```python
from build123d import *

# Parameters (mm, degrees)
SKETCH1_W           = 50.8
SKETCH1_H           = 25.4
SKETCH1_W_2         = 44.45
SKETCH1_H_2         = 19.05
BOSS_EXTRUDE1_DEPTH = 355.6
SKETCH2_R           = 3.3734375
CUT_EXTRUDE1_DEPTH  = 361.10715072


with BuildPart() as part:
    # Sketch1 → Boss-Extrude1 (new body)
    with BuildSketch(Plane(origin=(0, 0, 0), x_dir=(1, 0, 0), z_dir=(0, 1, 0))):
        with Locations((25.4, 12.7)):
            Rectangle(SKETCH1_W, SKETCH1_H)
        with Locations((25.4, 12.7)):
            Rectangle(SKETCH1_W_2, SKETCH1_H_2, mode=Mode.SUBTRACT)
    extrude(amount=BOSS_EXTRUDE1_DEPTH)

    # Sketch2 → Cut-Extrude1 (cut, through all)
    with BuildSketch(Plane(origin=(50.8, 0, 0), x_dir=(0, 0, -1), z_dir=(1, 0, 0))):
        with Locations((12.7, 12.7)):
            Circle(SKETCH2_R)
    cut_extrude1 = extrude(amount=-CUT_EXTRUDE1_DEPTH, mode=Mode.SUBTRACT)

    # Mirror1: Cut-Extrude1 across plane
    add(cut_extrude1.mirror(Plane.ZX.offset(177.8)), mode=Mode.SUBTRACT)


solid = part.part
```
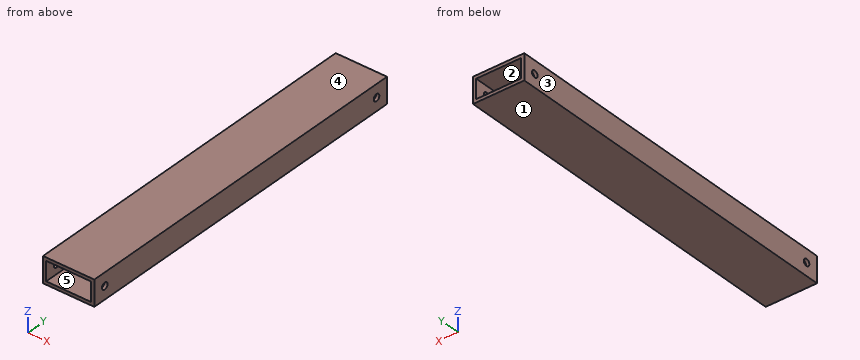
Check sheet for the modelled part. Datum: model origin and axes. Units: mm. Face numbers are marked on the shaded views. A direction names the side the tool comes from. Round coordinates to 2 decimals unless told otherwise and drop trailing zeros. Order: outer loops, then holes, each group sorted by start corner. A loop starts at its lowest first (then second) coordinate and runs counter-clockwise, first axis right, second up. Notation, with made-up numbers: (32.25, -18.5) - (81.25, -18.5) arc R22 cw to (81.25, -11.5) - close; hole circle Ø9 at (6.5, 19.5). An arc over 180 degrees is marked (long way). Answer as CSV lines item,"result". Start each with the question number.
1) Section check C-C (x = 22). Record the cut outline in (y, z) (3 decimals), then the cut area to 3 significant figures.
2) Scan lines: probe 1 along Y at (x, z) = (2, -12.7); probe 2 along X at (y, z) = (308, -11.5) (3 decimals); probe 3 along Z at (x, y) = (13.5, 321.5) (3 decimals). Record each from-to range of solid material in increasing order.
3) Tool access check on the marked faces 1 and 2. Record the directions out of +Z, -Z, +X, -X, +Y, -Y that give a thin tool (end or side, any length) a straight path to the whole face; none if there is none.
4) Section check B-B (z = -12.7). Record the cut outline in (x, y) (3 decimals).
5) Section check A-A (y = 12.7). Record the cut outline in (x, z) (3 decimals), then the cut area to 3 significant figures.
6) Draft check along X on the marked faces 3, 4 and 5. Enter one of: +X half, -X half, draft (parallel to the pull), parting line (faces both ways), or undercut.
Determined:
1,outline,"(0, -25.4) - (355.6, -25.4) - (355.6, -22.225) - (0, -22.225) - close; (0, -3.175) - (355.6, -3.175) - (355.6, 0) - (0, 0) - close"
1,area,"2,260 mm^2"
2,probe 1,"0 to 9.33, 16.07 to 339.53, 346.27 to 355.6"
2,probe 2,"0 to 3.175, 47.625 to 50.8"
2,probe 3,"-25.4 to -22.225, -3.175 to 0"
3,face 1,"-Z, +X, -X, +Y, -Y"
3,face 2,"+Y, -Y"
4,outline,"(0, 0) - (3.175, 0) - (3.175, 9.327) - (0, 9.327) - close; (0, 16.073) - (3.175, 16.073) - (3.175, 339.527) - (0, 339.527) - close; (0, 346.273) - (3.175, 346.273) - (3.175, 355.6) - (0, 355.6) - close; (47.625, 0) - (50.8, 0) - (50.8, 9.327) - (47.625, 9.327) - close; (47.625, 16.073) - (50.8, 16.073) - (50.8, 339.527) - (47.625, 339.527) - close; (47.625, 346.273) - (50.8, 346.273) - (50.8, 355.6) - (47.625, 355.6) - close"
5,outline,"(0, -25.4) - (50.8, -25.4) - (50.8, -16.073) - (47.625, -16.073) - (47.625, -22.225) - (3.175, -22.225) - (3.175, -16.073) - (0, -16.073) - close; (0, -9.327) - (3.175, -9.327) - (3.175, -3.175) - (47.625, -3.175) - (47.625, -9.327) - (50.8, -9.327) - (50.8, 0) - (0, 0) - close"
5,area,"401 mm^2"
6,face 3,"-X half"
6,face 4,"draft"
6,face 5,"undercut"
